Design review of the part built by this model. Coordinates are the model's own, in mm. A direction names the side the tool comes from. Coordinates: 2 decimals unless noted, no trailing zeros. Write each loop counter-clockwise with the first axis right and the second up, starting at its lowest first coordinate (ties: lowest second). Pieces come first, ordered by that corner, then holes. Notation, with made-up numbers: (54.25, 17) -> (70.25, 17) arc R23 ccw to (70.25, 48) -> close; hole circle Ø10 at (20, 36.5). An arc over 180 degrees is marked (long way). Answer in a Markdown table with one row per item. Add a question column.
Item 1: For faces 1 (the face through (-1.532, 37.185, 3.695)), 2 (the face through (-3.905, 3.944, -0.867)), 3 (the face through (0, 50, -3)), list the 3-axis set-ups (+Z, -Z, +X, -X, +Y, -Y) from which the entire face can be reached by the end or side of a thin tool; tool diameter is ignored.
Item 2: To check wall thickness, follow line 1 (X direction, y = 9.5, z = -0.25); line 2 (Z direction, x = 2.25, y = 12); line 3 (X direction, y = 28, z = -0.25). State the ranges of each line that lie inside material, in increasing order.
Item 3: Take a section at C-C, the plane y = 51. Write out the cut boundary in (x, z), and give its area (3 significant figures).
Item 4: Clearance check with flat-ended pins moving along their axes: P1, Ø3.5, axis at x = 0.5, y = 57, coming from the -Z side; P2, Ø1, axis at x = -1, y = 47.5, coming from the -Z side; P3, Ø3, axis at y = 36, z = 3.5, coming from the +X side. State where each tip first meets the part, or that it passes through.
Item 5: Take a section at B-B, the plane x = 0. Write out the cut boundary in (y, z).
Item 6: Take a section at D-D, the plane y = 18.5. Write out the cut boundary in (x, z), and give its area (3 significant figures).
Item 7: Take a section at A-A, the plane z = 0. Write out the cut boundary in (x, y), and give its area (3 significant figures).
from build123d import *

# Parameters (mm, degrees)
SKETCH1_R           = 4
BOSS_EXTRUDE1_DEPTH = 60
SKETCH2_R           = 5
BOSS_EXTRUDE2_DEPTH = 2
CHAMFER1_SIZE       = 1
CHAMFER1_SIZE_2     = 5
CUT_EXTRUDE1_START  = -10
CUT_EXTRUDE1_DEPTH  = 10


with BuildPart() as part:
    # Sketch1 → Boss-Extrude1 (new body)
    with BuildSketch(Plane(origin=(0, 0, 0), x_dir=(1, 0, 0), z_dir=(0, 1, 0))):
        with Locations(Location((0, 0, 0), (0, 0, 270))):
            Circle(SKETCH1_R)
    extrude(amount=BOSS_EXTRUDE1_DEPTH)

    # Sketch2 → Boss-Extrude2 (add)
    with BuildSketch(Plane(origin=(0, 8, 0), x_dir=(-1, 0, 0), z_dir=(0, -1, 0))):
        with Locations(Location((0, 0, 0), (0, 0, 90))):
            Circle(SKETCH2_R)
    extrude(amount=-BOSS_EXTRUDE2_DEPTH)

    # Chamfer1
    # the kernel refuses this chamfer: 5, 1 mm, written as the material it adds along each edge
    with BuildSketch(Plane(origin=(0, 10, 0), x_dir=(0, 0, 1), z_dir=(1, 0, 0))) as chamfer1_piece_1_section:
        Polygon((4 + CHAMFER1_SIZE, 0), (4, -CHAMFER1_SIZE_2), (4, 0), align=None)
    chamfer1_piece_1 = revolve(axis=Axis((0, 10, 0), (0, -1, 0)), mode=Mode.PRIVATE)
    chamfer1_piece_1 = chamfer1_piece_1 & Plane(origin=(0, 12.589419048, 0), x_dir=(0, 0, -1), z_dir=(0, -1, 0)) * Cylinder(5, 20, mode=Mode.PRIVATE)
    add(chamfer1_piece_1)

    # Sketch3 → Cut-Extrude1 (cut)
    with BuildSketch(Plane(origin=(0, 60, 0), x_dir=(1, 0, 0), z_dir=(0, 1, 0)).offset(CUT_EXTRUDE1_START)):
        with BuildLine():
            Line((-3.307189139, 2.25), (3.307189139, 2.25))
            ThreePointArc((3.307189139, 2.25), (0, 4), (-3.307189139, 2.25))
        make_face()
    extrude(amount=CUT_EXTRUDE1_DEPTH, mode=Mode.SUBTRACT)


solid = part.part
Answers:
| question | item | result |
|---|---|---|
| 1 | face 1 | +Y |
| 1 | face 2 | -Y |
| 1 | face 3 | -Z, +X, -X, +Y |
| 2 | line 1 | x = -4.99 to 4.99 |
| 2 | line 2 | z = -4.01 to 4.01 |
| 2 | line 3 | x = -3.99 to 3.99 |
| 3 | outline | (-3.31, -2.25) -> (3.31, -2.25) arc R4 ccw (long way) to start |
| 3 | area | 42.1 mm^2 |
| 4 | P1 | stops at z = -2.25 |
| 4 | P2 | stops at z = -3.97 |
| 4 | P3 | stops at x = 3.46 |
| 5 | outline | (0, -4) -> (8, -4) -> (8, -5) -> (10, -5) -> (15, -4) -> (50, -4) -> (50, -2.25) -> (60, -2.25) -> (60, 4) -> (15, 4) -> (10, 5) -> (8, 5) -> (8, 4) -> (0, 4) -> close |
| 6 | outline | circle Ø8 at (0, 0) |
| 6 | area | 50.3 mm^2 |
| 7 | outline | (-5, 8) -> (-4, 8) -> (-4, 0) -> (4, 0) -> (4, 8) -> (5, 8) -> (5, 10) -> (4, 15) -> (4, 60) -> (-4, 60) -> (-4, 15) -> (-5, 10) -> close |
| 7 | area | 489 mm^2 |
